Check sheet for the modelled part. Datum: model origin and axes. Units: mm. A direction names the side the tool comes from. Round coordinates to 2 decimals unless told otherwise and drop trailing zeros. Order: outer loops, then holes, each group sorted by start corner. A loop starts at its lowest first (then second) coordinate and runs counter-clockwise, first axis right, second up. Notation, with made-up numbers: M -14,13.25 L 41,13.25 A27 cw 41,50.25 Z; hole C 24,26 d3. An arc over 180 degrees is marked long. One line per item, written item: value. Start each with the question number.
(1) Thickness scan on L1, parallel to Z at x = 0, y = 1.7; L2, parallel to Y at x = 6.5, z = -1.25; L3, parallel to X at y = 7, z = 0. Record the ranges inside material, lowest first.
(2) Cross-section at D-D, the plane y = 27. Enter the section's corners in (x, z).
(3) Release check for a two-part mould opening along X. For faces 5 (the face through (-0.11, 15.16, 3.15)), 6 (the face through (0, 31.5, 0)), 7 (the face through (-0.63, 0.49, 6.82)) record: released by +X, released by -X, zero draft, split by the parting line, or undercut.
(4) Access from +Z, -Z, +X, -X, +Y, -Y to the whole of each face (thin tool, end or side, straight path). Record for faces 1 (the face through (0, 8.5, -3)), 2 (the face through (0, 20, -2.422)), 3 (the face through (0, 5, 0)), 4 (the face through (0.63, 0.49, -6.82)).
(5) Depth check by flat-ended pin: pin 1 Ø4 at (x, y) = (0, 7) entering from +Z; pin 2 Ø8 at (x, z) = (0, 0) entering from -Y; pin 3 Ø3 at (x, z) = (-0.37, 7.99) entering from +Y; pin 4 Ø2 at (x, z) = (7.99, 0.37) entering from -Y. Enter the tip coordinate at first touch or a pass-through.
(6) Cross-section at C-C, the plane y = 13. Enter the section's corners in (x, z).
(7) Cross-section at A-A, the plane z = 0. Count the separate pieces of the cut face and the enclosed holes in it, and give its area (3 significant figures).
from build123d import *

# Parameters (mm, degrees)
ESQUISSE3_W                  = 6.57785754
ESQUISSE3_H                  = 1.386048805
ENL_V_MAT_EXTRU_1_DEPTH      = 23
M2_CLEARANCE_HOLE1_D         = 2.4
M2_CLEARANCE_HOLE1_DEPTH     = 1.001
R_P_TITION_CIRCULAIRE1_COUNT = 4
FILLET1_R                    = 0.5


with BuildPart() as part:
    # Esquisse2 → Révolution2 (revolve)
    with BuildSketch(Plane.XY):
        Polygon((0, 31.5), (3, 31.5), (3, 21.5), (3.15, 21.5), (3.15, 8.5), (6.2, 8.5), (6.2, 3), (6.2, 1), (10, 1), (10, 0), (4.5, 0), (4.5, 5), (0, 5), align=None)
    revolve(axis=Axis((0, 5, 0), (0, 1, 0)))

    # Esquisse3 → Enlèv. mat.-Extru.1 (cut)
    with BuildSketch(Plane(origin=(0, 31.5, 0), x_dir=(1, 0, 0), z_dir=(0, 1, 0))):
        with Locations((-0.352413472, 3.114928535)):
            Rectangle(ESQUISSE3_W, ESQUISSE3_H)
    extrude(amount=-ENL_V_MAT_EXTRU_1_DEPTH, mode=Mode.SUBTRACT)

    # M2 Clearance Hole1
    with Locations(Plane(origin=(0, 1, 0), x_dir=(1, 0, 0), z_dir=(0, 1, 0))):
        with Locations((0.371303159, 7.991378727)):
            m2_clearance_hole1 = Hole(M2_CLEARANCE_HOLE1_D / 2, depth=M2_CLEARANCE_HOLE1_DEPTH)

    # Répétition circulaire1: M2 Clearance Hole1 ×4 about axis
    r_p_tition_circulaire1_axis = Axis((0, 0, 0), (0, 1, 0))
    for i in range(1, R_P_TITION_CIRCULAIRE1_COUNT):
        add(m2_clearance_hole1.rotate(r_p_tition_circulaire1_axis, i * 360 / R_P_TITION_CIRCULAIRE1_COUNT), mode=Mode.SUBTRACT)

    # Fillet1
    fillet1_edges = [part.edges().sort_by_distance(p)[0] for p in [
        (-6.2, 1, 0),
        (-6.2, 8.5, 0),
        (0, 8.5, 3.15),
    ]]
    fillet(fillet1_edges, radius=FILLET1_R)


solid = part.part
Values found:
1. L1: -6.2 to -4.5, 4.5 to 6.2
1. L2: 0 to 1.01
1. L3: -6.2 to 6.2
2. outline: M -1.77,-2.42 L 1.77,-2.42 A3 ccw long Z
3. face 5: split by the parting line
3. face 6: zero draft
3. face 7: undercut
4. face 1: +Y
4. face 2: -Z, +X, -X, +Y
4. face 3: -Y
4. face 4: +Y, -Y
5. pin 1: z = 6.2
5. pin 2: y = 5
5. pin 3: y = 1.04
5. pin 4: through
6. outline: M -2.01,-2.42 L 2.01,-2.42 A3.15 ccw long Z
7. separate pieces: 3
7. enclosed holes: 0
7. area: 205 mm^2
